from build123d import *

# Parameters (mm, degrees)
F0_W     = 64.77
F0_H     = 44.958
F1_DEPTH = 26.543
F2_W     = 3.9624
F2_H     = 32.258
F2_W_2   = 17.018
F2_H_2   = 20.193
F3_DEPTH = 26.544
F4_W     = 6.8494506996
F4_H     = 2.032
F5_DEPTH = 47.753
F7_DEPTH = 11.7856
F8_R     = 5.1308
F9_DEPTH = 31.75


with BuildPart() as f1:
    # F0 (on Top) → F1 (new body)
    with BuildSketch(Plane.XY):
        Rectangle(F0_W, F0_H)
    extrude(amount=F1_DEPTH)

    # F2 (on face) → F3 (cut, through all)
    with BuildSketch(Plane.XY.offset(26.543)):
        with Locations((-30.4038, 6.35)):
            Rectangle(F2_W, F2_H)
        with Locations((23.876, 12.3825)):
            Rectangle(F2_W_2, F2_H_2)
    extrude(amount=-F3_DEPTH, mode=Mode.SUBTRACT)

    # F4 (on face) → F5 (cut, through all)
    with BuildSketch(Plane.YZ.offset(15.367)):
        with BuildLine():
            Line((7.3680459394, 24.511), (7.3680459394, 14.8504350737))
            ThreePointArc((7.3680459394, 14.8504350737), (10.8413795833, 11.3033136722), (14.2174966391, 14.9430870806))
            Line((14.2174966391, 14.9430870806), (14.2174966391, 24.511))
            Line((14.2174966391, 24.511), (7.3680459394, 24.511))
        make_face()
        Polygon((2.7917712892, 24.511), (7.3680459394, 24.511), (7.3680459394, 26.543), (14.2174966391, 26.543), (14.2174966391, 24.511), (18.7937712892, 24.511), (18.7937712892, 28.575), (2.7917712892, 28.575), align=None)
        with Locations((10.7927712892, 25.527)):
            Rectangle(F4_W, F4_H)
    extrude(amount=-F5_DEPTH, mode=Mode.SUBTRACT)

    # F6 (on face) → F7 (cut)
    with BuildSketch(Plane.XY.offset(26.543)):
        with BuildLine():
            Line((22.5425, -22.479), (22.5425, -8.8392))
            ThreePointArc((22.5425, -8.8392), (14.5724547472, -0.9017667211), (6.6677668834, -8.9042899584))
            Line((6.6677668834, -8.9042899584), (6.6677668834, -10.5686287108))
            Line((6.6677668834, -10.5686287108), (5.5927410722, -10.5686287108))
            Line((5.5927410722, -10.5686287108), (-6.8503879466, -3.5582287108))
            ThreePointArc((-6.8503879466, -3.5582287108), (-15.6017772044, -1.421651907), (-20.7137, -8.8392))
            Line((-20.7137, -8.8392), (-20.7137, -22.479))
            Line((-20.7137, -22.479), (22.5425, -22.479))
        make_face()
    extrude(amount=-F7_DEPTH, mode=Mode.SUBTRACT)

    # F8 (on face) → F9 (cut)
    with BuildSketch(Plane.YZ.offset(32.385)):
        with Locations((-7.2898, 7.9248)):
            Circle(F8_R)
    extrude(amount=-F9_DEPTH, mode=Mode.SUBTRACT)


solid = f1.part
Verification items for the finished model (mm, model axes). A direction names the side the tool comes from. Give positions to 0.01 mm unless a question says otherwise; leave off trailing zeros. Order: outer loops, then holes, each group sorted by start corner. A loop starts at its lowest first (then second) coordinate and runs counter-clockwise, first axis right, second up. Notation, with made-up numbers: M 60,-22 L 88,-22 A11 cw 88,-15 Z; hole C 2,-37 d4. An arc over 180 degrees is marked long. Use one line per item in the form item = value. Start each with the question number.
Q1. Section check C-C (x = 20). Enter the section's corners in (y, z), then the cut area to 3 significant figures.
Q2. Section check A-A (z = 20). Enter the section's corners in (x, y) (1 decimal), then the cut area to 3 significant figures.
Q3. Scan lines: line 1 along Z through (x, y) = (-14, 18); line 2 along X through (y, z) = (-10.5, 20.25) (1 decimal); line 3 along Z through (x, y) = (-9, -9.5). Record each from-to range of solid material in increasing order. Write a range as [from, to].
Q4. Mould release check, pull along Y, two halves, no side actions. Record for faces 4 (the flat face through (-7, 22.479, 13)), 5 (the flat face through (-28.423, 6, 13)), 6 (the cylindrical face through (16.732, -11.071, 11.392)): +Y half, -Y half, draft (parallel to the pull), parting line (faces both ways), or undercut.
Q5. Section check D-D (x = -21.5). Enter the section's corners in (y, z) (1 decimal), then the cut area to 3 significant figures.
Q6. Go/stop test with flat-tipped pins: pin 1 Ø3 at (y, z) = (10.5, 11.5) entering from -X; pin 2 Ø1.2 at (x, z) = (6.5, 18) entering from -Y; pin 3 Ø5 at (x, y) = (-15.5, 9.5) entering from +Z. Record where each tip stops, or that it passes through.
Q7. Section check B-B (y = -14). Enter the section's corners in (x, z) (1 decimal), then the cut area to 3 significant figures.
Q8. Access from +Z, -Z, +X, -X, +Y, -Y to the whole of each face (thin tool, end or side, straight path). Record for faces 1 (the flat face through (-6, 2.792, 26)), 2 (the flat face through (-0.542, -7.113, 20.733)), 3 (the flat face through (-32.385, -16, 13)).
Evaluation:
q1.outline = M -22.48,0 L 2.29,0 L 2.29,26.54 L -3.02,26.54 L -3.02,14.76 L -22.48,14.76 Z; hole C -7.29,7.92 d10.26
q1.area = 345 mm2
q2.outline = M -32.4,-22.5 L -20.7,-22.5 L -20.7,-8.8 A7.9 cw -6.9,-3.6 L 5.6,-10.6 L 6.7,-10.6 L 6.7,-8.9 A7.9 cw long 22.5,-8.8 L 22.5,-22.5 L 32.4,-22.5 L 32.4,2.3 L 15.4,2.3 L 15.4,7.4 L -28.4,7.4 L -28.4,-9.8 L -32.4,-9.8 Z; M -28.4,14.2 L 15.4,14.2 L 15.4,22.5 L -28.4,22.5 Z
q2.area = 1,340 mm2
q3.line_1 = [0, 24.51]
q3.line_2 = [-32.4, -20.7], [5.5, 6.7], [22.5, 32.4]
q3.line_3 = [0, 14.76]
q4.face_4 = +Y half
q4.face_5 = draft
q4.face_6 = undercut
q5.outline = M -22.5,0 L 22.5,0 L 22.5,26.5 L 18.8,26.5 L 18.8,24.5 L 14.2,24.5 L 14.2,14.9 A3.4 cw long 7.4,14.9 L 7.4,24.5 L 2.8,24.5 L 2.8,26.5 L -22.5,26.5 Z
q5.area = 1,080 mm2
q6.pin_1 = -28.42
q6.pin_2 = -10.57
q6.pin_3 = 24.51
q7.outline = M -32.4,0 L 32.4,0 L 32.4,26.5 L 22.5,26.5 L 22.5,14.8 L -20.7,14.8 L -20.7,26.5 L -32.4,26.5 Z
q7.area = 1,210 mm2
q8.face_1 = +Z, +X, -X
q8.face_2 = +Z, -Y
q8.face_3 = +Z, -Z, -X, +Y, -Y
